The listing builds one solid part. Answer for the finished solid, in the listing's coordinates (mm). Face numbers are marked on the shaded views. Round coordinates to 2 decimals unless told otherwise and drop trailing zeros. Order: outer loops, then holes, each group sorted by start corner. A loop starts at its lowest first (then second) coordinate and runs counter-clockwise, first axis right, second up. Notation, with made-up numbers: (-33.5, 53.25) - (19.5, 53.25) arc R6 ccw to (19.5, 59.25) - close; hole circle Ø6 at (-10, 87.25). An arc over 180 degrees is marked (long way). One line per item, written item: value. Start each with the question number.
1. Section D-D, the plane x = -7 is taken. Give the vertices of the cut face in (y, z).
2. Section A-A, the plane y = -0.4 is taken. Give the vertices of the cut face in (x, z), then the cut area to 3 significant figures.
3. For a pull along Z with two mould halves and no side action, classify the marked faces 1 and 2 as released by +Z, released by -Z, zero draft, split by the parting line, or undercut.
4. Flat-ended cylindrical pins translate along their axes: P1, Ø3, axis at x = -36, z = -40.99, coming from the -Y side; P2, Ø0.8, axis at x = 12.5, y = -0.5, coming from the +Z side; P3, Ø0.5, axis at y = -0.5, z = -41, coming from the -X side; P4, Ø2, axis at x = 36, z = 41.01, coming from the +Y side. Find the tip coordinate at first contact, or state that the pin passes through.
5. Section B-B, the plane z = 15 is taken. Give the vertices of the cut face in (x, y), then the cut area to 3 significant figures.
6. Straight lines are drawn through the part: line 1 (X direction, y = -0.1, z = 3.5); line 2 (Z direction, x = -27, y = -0.5); line 3 (Y direction, x = 16, z = -33.5). For each, find the intervals that lie inside material, in ascending order.
7. Section C-C, the plane x = 21 is taken. Give the vertices of the cut face in (y, z), then the cut area to 3 significant figures.
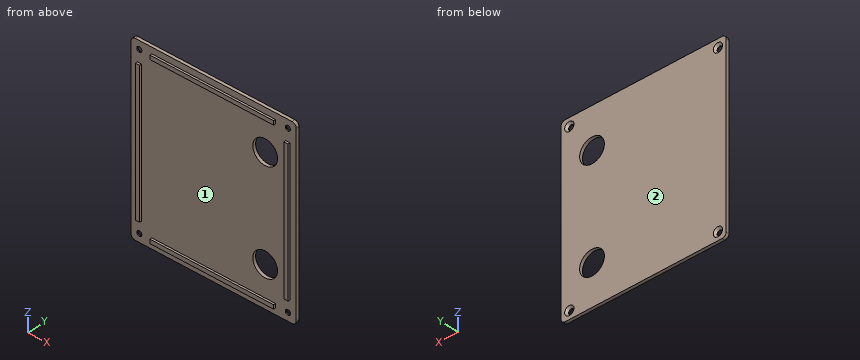
Autodesk Fusion 360 part; units mm, degrees
sketch "Skizze1" plane through (0, 0, 0) normal (0, 1, 0) x (1, 0, 0)
  line L0 (-39.9994, 44.9914) -> (40.0006, 44.9914)
  line L1 (40.0006, 44.9914) -> (40.0006, -45.0086)
  line L2 (40.0006, -45.0086) -> (-39.9994, -45.0086)
  line L3 (-39.9994, -45.0086) -> (-39.9994, 44.9914)
  circle A0 centre (-35.9994, 40.9914) radius 1.25
  circle A1 centre (36.0006, 40.9914) radius 1.25
  circle A2 centre (36.0006, -41.0086) radius 1.25
  circle A3 centre (-35.9994, -41.0086) radius 1.25
  circle A4 centre (25.0006, 24.9914) radius 6
  circle A5 centre (25.0006, -25.0086) radius 6
  dimension "d1" = 80
  dimension "d2" = 90
  dimension "d3" = 2.5
  dimension "d4" = 4
  dimension "d5" = 4
  dimension "d6" = 2.5
  dimension "d7" = 4
  dimension "d8" = 4
  dimension "d9" = 2.5
  dimension "d10" = 4
  dimension "d11" = 4
  dimension "d12" = 2.5
  dimension "d13" = 4
  dimension "d14" = 4
  dimension "d39" = 12
  dimension "d40" = 12
  dimension "d41" = 15
  dimension "d42" = 20
  dimension "d43" = 15
  dimension "d44" = 20
extrude "Extrusion1" add sketch "Skizze1" along normal blind 1.5
fillet "Abrundung1" radius 2 1 edges at (-39.9994, 0.75, 45.0086)
fillet "Abrundung1" radius 2 1 edges at (40.0006, 0.75, 45.0086)
fillet "Abrundung1" radius 2 1 edges at (-39.9994, 0.75, -44.9914)
fillet "Abrundung1" radius 2 1 edges at (40.0006, 0.75, -44.9914)
chamfer "Fase1" distance 1 angle 45 1 edges at (-37.1648, 1.5, -41.4434)
chamfer "Fase1" distance 1 angle 45 1 edges at (34.8352, 1.5, -41.4434)
chamfer "Fase1" distance 1 angle 45 1 edges at (-37.1648, 1.5, 40.5566)
chamfer "Fase1" distance 1 angle 45 1 edges at (34.8352, 1.5, 40.5566)
sketch "Skizze3" plane through (0, 0, 0) normal (0, -1, 0) x (1, 0, 0)
  arc A0 (38.0006, -44.9914) -> (40.0006, -42.9914) centre (38.0006, -42.9914) ccw
  line L0 (40.0006, -42.9914) -> (40.0006, 43.0086)
  arc A1 (40.0006, 43.0086) -> (38.0006, 45.0086) centre (38.0006, 43.0086) ccw
  line L1 (38.0006, 45.0086) -> (-37.9994, 45.0086)
  arc A2 (-37.9994, 45.0086) -> (-39.9994, 43.0086) centre (-37.9994, 43.0086) ccw
  line L2 (-39.9994, 43.0086) -> (-39.9994, -42.9914)
  arc A3 (-39.9994, -42.9914) -> (-37.9994, -44.9914) centre (-37.9994, -42.9914) ccw
  line L3 (-37.9994, -44.9914) -> (38.0006, -44.9914)
  circle A4 centre (-35.9994, -40.9914) radius 1.25
  circle A5 centre (36.0006, 41.0086) radius 1.25
  circle A6 centre (36.0006, -40.9914) radius 1.25
  circle A7 centre (-35.9994, 41.0086) radius 1.25
  line L4 (-36.9994, 35) -> (-34.9994, 35)
  line L5 (-34.9994, 35) -> (-34.9994, -35)
  line L6 (-34.9994, -35) -> (-36.9994, -35)
  line L7 (-36.9994, -35) -> (-36.9994, 35)
  line L8 (-30, 42.0086) -> (30, 42.0086)
  line L9 (30, 42.0086) -> (30, 40.0086)
  line L10 (30, 40.0086) -> (-30, 40.0086)
  line L11 (-30, 40.0086) -> (-30, 42.0086)
  line L12 (37.0006, 35) -> (35.0006, 35)
  line L13 (35.0006, 35) -> (35.0006, -35)
  line L14 (35.0006, -35) -> (37.0006, -35)
  line L15 (37.0006, -35) -> (37.0006, 35)
  line L16 (30, -41.9914) -> (-30, -41.9914)
  line L17 (-30, -41.9914) -> (-30, -39.9914)
  line L18 (-30, -39.9914) -> (30, -39.9914)
  line L19 (30, -39.9914) -> (30, -41.9914)
  circle A8 centre (25.0006, -24.9914) radius 6
  circle A9 centre (25.0006, 25.0086) radius 6
  dimension "d29" = 2
  dimension "d30" = 2
  dimension "d31" = 2
  dimension "d32" = 2
  dimension "d33" = 3
  dimension "d34" = 3
  dimension "d35" = 3
  dimension "d36" = 3
extrude "Extrusion2" add sketch "Skizze3" along normal blind 1 contours L4 L5 L6 L7 | L8 L9 L10 L11 | L12 L13 L14 L15 | L16 L17 L18 L19
Answer list:
1. outline: (-1, -41.99) - (0, -41.99) - (0, -44.99) - (1.5, -44.99) - (1.5, 45.01) - (0, 45.01) - (0, 42.01) - (-1, 42.01) - (-1, 40.01) - (0, 40.01) - (0, -39.99) - (-1, -39.99) - close
2. outline: (-37, -35) - (-35, -35) - (-35, 35) - (-37, 35) - close; (-30, -41.99) - (30, -41.99) - (30, -39.99) - (-30, -39.99) - close; (-30, 40.01) - (30, 40.01) - (30, 42.01) - (-30, 42.01) - close; (35, -35) - (37, -35) - (37, 35) - (35, 35) - close
2. area: 520 mm²
3. face 1: undercut
3. face 2: zero draft
4. P1: stops at y = 0
4. P2: stops at z = 42.01
4. P3: stops at x = -30
4. P4: passes through
5. outline: (-40, 0) - (-37, 0) - (-37, -1) - (-35, -1) - (-35, 0) - (35, 0) - (35, -1) - (37, -1) - (37, 0) - (40, 0) - (40, 1.5) - (-40, 1.5) - close
5. area: 124 mm²
6. line 1: x = -37 to -35, 35 to 37
6. line 2: z = -41.99 to -39.99, 40.01 to 42.01
6. line 3: y = 0 to 1.5
7. outline: (-1, -41.99) - (0, -41.99) - (0, -44.99) - (1.5, -44.99) - (1.5, -29.46) - (0, -29.46) - (0, -39.99) - (-1, -39.99) - close; (-1, 40.01) - (0, 40.01) - (0, 29.48) - (1.5, 29.48) - (1.5, 45.01) - (0, 45.01) - (0, 42.01) - (-1, 42.01) - close; (0, -20.52) - (1.5, -20.52) - (1.5, 20.54) - (0, 20.54) - close
7. area: 112 mm²
